Geometry: final body of the model. Coordinates: model frame, mm. Give positions to 0.01 mm unless a question says otherwise; leave off trailing zeros. Write each loop counter-clockwise with the first axis right and the second up, starting at its lowest first coordinate (ties: lowest second). Pieces come first, ordered by that corner, then holes.
Q1. Pin query (flat end, axial travel): pin 1 (1.2 mm diameter, centred on x = -1.5, y = 0, fed in from -Z); pin 2 (2 mm diameter, centred on x = 29, y = -0.5, fed in from -Z); pin 3 (3 mm diameter, centred on y = 2.5, z = -4.5, fed in from +X); pin 4 (4 mm diameter, centred on x = 30.5, z = -3, fed in from +Y). Return the tip coordinate at first contact, or that it passes through.
Q2. Cut plane C-C on x = 26. Return the cut outline in (y, z), plus the area to 3 significant figures.
Q3. Cut plane B-B on z = -0.5. Return the cut outline in (x, y), plus the area to 3 significant figures.
Q4. Cut plane A-A on y = 0. Return the cut outline in (x, z).
Q5. Line query: L1, parallel to X at y = -4, z = -4.5; L2, parallel to Z at x = 27.5, y = -0.5; L3, parallel to Y at x = 32, z = 1. Output: solid intervals per line, ascending.
Q6. Cut plane D-D on y = 3.25. Return the cut outline in (x, z), plus the area to 3 significant figures.
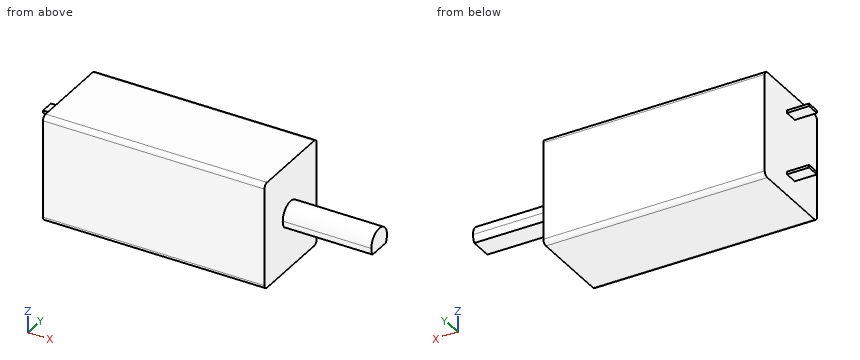
```python
from build123d import *

# Parameters (mm, degrees)
EXTRUDE_1_DEPTH = 25
EXTRUDE_2_DEPTH = 10
SKETCH_3_W      = 0.3
SKETCH_3_H      = 1.5
EXTRUDE_3_DEPTH = 2.5


with BuildPart() as part:
    # 草图1 → 凸台-拉伸1 (new body)
    with BuildSketch(Plane(origin=(0, 0, 0), x_dir=(0, 0, -1), z_dir=(1, 0, 0))):
        with BuildLine():
            Line((-5.5, 5), (5.5, 5))
            ThreePointArc((5.5, 5), (5.853553391, 4.853553391), (6, 4.5))
            Line((6, 4.5), (6, -4.5))
            ThreePointArc((6, -4.5), (5.853553391, -4.853553391), (5.5, -5))
            Line((5.5, -5), (-5.5, -5))
            ThreePointArc((-5.5, -5), (-5.853553391, -4.853553391), (-6, -4.5))
            Line((-6, -4.5), (-6, 4.5))
            ThreePointArc((-6, 4.5), (-5.853553391, 4.853553391), (-5.5, 5))
        make_face()
    extrude(amount=EXTRUDE_1_DEPTH)

    # 草图2 → 凸台-拉伸2 (add)
    with BuildSketch(Plane(origin=(25, 0, 0), x_dir=(0, 0, -1), z_dir=(1, 0, 0))):
        with BuildLine():
            ThreePointArc((0.829156198, 1.25), (0.433012702, 1.436140662), (0, 1.5))
            Line((0, 1.5), (0, -1.5))
            ThreePointArc((0, -1.5), (0.433012702, -1.436140662), (0.829156198, -1.25))
            Line((0.829156198, -1.25), (0.829156198, 1.25))
        make_face()
        with BuildLine():
            Line((0, -1.5), (0, 1.5))
            ThreePointArc((0, 1.5), (-1.5, 0), (0, -1.5))
        make_face()
    extrude(amount=EXTRUDE_2_DEPTH)

    # 草图3 → 凸台-拉伸3 (add)
    with BuildSketch(Plane.ZY):
        with Locations((-3.5, 0)):
            Rectangle(SKETCH_3_W, SKETCH_3_H)
        with Locations((3.5, 0)):
            Rectangle(SKETCH_3_W, SKETCH_3_H)
    extrude(amount=EXTRUDE_3_DEPTH)


solid = part.part
```
Data:
1. pin 1: stops at z = -3.65
1. pin 2: stops at z = -0.83
1. pin 3: stops at x = 25
1. pin 4: passes through
2. outline: (-1.25, -0.83) - (1.25, -0.83) arc R1.5 ccw (long way) to start
2. area: 5.89 mm2
3. outline: (0, -5) - (25, -5) - (25, -1.41) - (35, -1.41) - (35, 1.41) - (25, 1.41) - (25, 5) - (0, 5) - close
3. area: 278 mm2
4. outline: (-2.5, -3.65) - (0, -3.65) - (0, -6) - (25, -6) - (25, -0.83) - (35, -0.83) - (35, 1.5) - (25, 1.5) - (25, 6) - (0, 6) - (0, 3.65) - (-2.5, 3.65) - (-2.5, 3.35) - (0, 3.35) - (0, -3.35) - (-2.5, -3.35) - close
5. L1: x = 0 to 25
5. L2: z = -0.83 to 1.41
5. L3: y = -1.12 to 1.12
6. outline: (0, -6) - (25, -6) - (25, 6) - (0, 6) - close
6. area: 300 mm2
